The listing builds one solid part. Answer for the finished solid, in the listing's coordinates (mm). Face numbers are marked on the shaded views. Give positions to 0.01 mm unless a question says otherwise; leave off trailing zeros. Use a Markdown table: item, result. Add a question column.
1) Flat-ended cylindrical pins translate along their axes: pin 1 (5 mm diameter, centred on x = -2.5, y = -17, fed in from -Z); pin 2 (1 mm diameter, centred on x = -4.5, z = -4, fed in from -Y); pin 3 (10 mm diameter, centred on y = -43.5, z = -26.5, fed in from +X). Find the tip coordinate at first contact, or state that the pin passes through.
2) The mould has two halves that part along X. Classify the marked faces 1, 2 and 3: released by +X, released by -X, zero draft, split by the parting line, or undercut.
3) Straight lines are drawn through the part: line 1 (Y direction, x = -6.75, z = -1); line 2 (X direction, y = -55.5, z = -13); line 3 (X direction, y = -52, z = -4). For each, find the intervals that lie inside material, in ascending order.
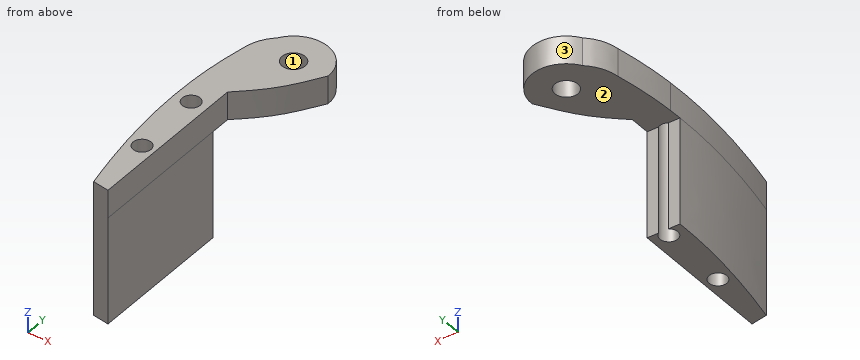
from build123d import *

# Parameters (mm, degrees)
SKETCH1_R           = 2.9
BOSS_EXTRUDE1_DEPTH = 7
BOSS_EXTRUDE2_DEPTH = 26.812432
SKETCH3_R           = 2.25
CUT_EXTRUDE1_DEPTH  = 81.286678341


with BuildPart() as part:
    # Sketch1 → Boss-Extrude1 (new body)
    with BuildSketch(Plane.XY):
        with BuildLine():
            Line((-14.153385189, -69.716871134), (-10.039841479, -70.438427685))
            Line((-10.039841479, -70.438427685), (-10.231600818, -28.548135162))
            add(Edge.make_bspline(
                [(3.150526507, -12), (1.121426745, -15.448537633), (-2.522354698, -21.641292501), (-7.864373324, -26.42729642), (-10.231600818, -28.548135162)],
                knots=[0, 0, 0, 0, 0.556866484, 1, 1, 1, 1], degree=3))
            ThreePointArc((3.150526507, -12), (-3.18362895, -3.611112101), (-12.986183722, -7.406488955))
            add(Edge.make_bspline(
                [(-16.663916234, -14.630806425), (-16.157795835, -10.23676377), (-12.986183722, -7.406488955)],
                knots=[0, 0, 0, 1, 1, 1], degree=2))
            add(Edge.make_bspline(
                [(-16.663916234, -14.630806425), (-17.667702323, -19.881251045), (-18.220131563, -25.189037493), (-18.401311599, -30.514562532)],
                knots=[0, 0, 0, 0, 0.288118642, 0.288118642, 0.288118642, 0.288118642], degree=3))
            add(Edge.make_bspline(
                [(-18.401311599, -30.514562532), (-18.848969857, -43.672829442), (-17.03022033, -56.93938717), (-14.153385189, -69.716871134)],
                knots=[0.288118642, 0.288118642, 0.288118642, 0.288118642, 1, 1, 1, 1], degree=3))
        make_face()
        with Locations((-5.571628032, -12)):
            Circle(SKETCH1_R, mode=Mode.SUBTRACT)
    extrude(amount=-BOSS_EXTRUDE1_DEPTH)

    # Sketch2 → Boss-Extrude2 (add)
    with BuildSketch(Plane(origin=(0, 0, -7), x_dir=(-1, 0, 0), z_dir=(0, 0, -1))):
        with BuildLine():
            Line((10.039841479, -70.438427685), (14.153385189, -69.716871134))
            add(Edge.make_bspline(
                [(14.153385189, -69.716871134), (16.794208846, -57.987633874), (18.543433317, -45.846277061), (18.466393507, -33.754875992)],
                knots=[0.346520381, 0.346520381, 0.346520381, 0.346520381, 1, 1, 1, 1], degree=3))
            Line((18.466393507, -33.754875992), (15.532606101, -33.741446123))
            ThreePointArc((15.532606101, -33.741446123), (14.280806546, -37.867902739), (13.066837656, -33.730158684))
            Line((13.066837656, -33.730158684), (10.207939206, -33.717071631))
            Line((10.207939206, -33.717071631), (10.039841479, -70.438427685))
        make_face()
    extrude(amount=BOSS_EXTRUDE2_DEPTH)

    # Sketch3 → Cut-Extrude1 (cut, through all)
    with BuildSketch(Plane.XY):
        with Locations((-14.291106163, -35.617926313)):
            Circle(SKETCH3_R)
        with Locations((-13.459661862, -53.850312066)):
            Circle(SKETCH3_R)
    extrude(amount=-CUT_EXTRUDE1_DEPTH, mode=Mode.SUBTRACT)


solid = part.part
The answers:
| question | item | result |
|---|---|---|
| 1 | pin 1 | z = -7 |
| 1 | pin 2 | y = -23.61 |
| 1 | pin 3 | x = -10.14 |
| 2 | face 1 | undercut |
| 2 | face 2 | zero draft |
| 2 | face 3 | split by the parting line |
| 3 | line 1 | -25.36 to -14.65, -9.35 to -3.36 |
| 3 | line 2 | -16.83 to -14.99, -11.93 to -10.11 |
| 3 | line 3 | -17.31 to -14.74, -12.18 to -10.12 |
